The model under review builds one solid part; all positions refer to its coordinate system, in mm. A direction names the side the tool comes from. Coordinates: 2 decimals unless noted, no trailing zeros. Order: outer loops, then holes, each group sorted by start corner. A loop starts at its lowest first (then second) coordinate and runs counter-clockwise, first axis right, second up. Notation, with made-up numbers: M 79.25,70 L 97.25,70 A28 ccw 97.25,99 Z; hole C 26,16 d7. An arc over 180 degrees is marked long. Answer in a Markdown table with one row per item.
from build123d import *

# Parameters (mm, degrees)
F0_W     = 4.25
F0_H     = 4.25
F1_DEPTH = 5
F3_START = 2
F3_DEPTH = 4
F4_START = -2
F4_DEPTH = 4


# Not quite as in the source:
# - a feature names something its author has since deleted; it is built from what else it names


with BuildPart() as f1:
    # F0 (on Top) → F1 (new body, symmetric)
    with BuildSketch(Plane.XY):
        with BuildLine():
            Line((10.48, -5), (10.48, 5))
            Line((10.48, 5), (0.8137170322, 5))
            ThreePointArc((0.8137170322, 5), (1.6624848855, 2.5140482951), (1.95, -0.0970238614))
            ThreePointArc((1.95, -0.0970238614), (1.6852450978, -2.6038191253), (0.9026629175, -5))
            Line((0.9026629175, -5), (10.48, -5))
        make_face()
        with Locations((5.23, -0.25)):
            Rectangle(F0_W, F0_H, mode=Mode.SUBTRACT)
        with BuildLine():
            ThreePointArc((1.95, -0.0970238614), (1.6624848855, 2.5140482951), (0.8137170322, 5))
            Line((0.8137170322, 5), (0.48, 5))
            Line((0.48, 5), (0.48, -5))
            Line((0.48, -5), (0.9026629175, -5))
            ThreePointArc((0.9026629175, -5), (1.6852450978, -2.6038191253), (1.95, -0.0970238614))
        make_face()
        with BuildLine():
            Line((0.48, 5), (0.8137170322, 5))
            ThreePointArc((0.8137170322, 5), (-11.6370433083, 11.7975670747), (-21.8700390085, 1.9734055232))
            Line((-21.8700390085, 1.9734055232), (-20.3438487537, 1.9734055232))
            ThreePointArc((-20.3438487537, 1.9734055232), (-9.0096663788, 10.3513112192), (0.45, -0.0970238614))
            ThreePointArc((0.45, -0.0970238614), (-9.0810805838, -10.5522232935), (-20.3711800314, -2.0265944768))
            Line((-20.3711800314, -2.0265944768), (-21.89384892, -2.0265944768))
            ThreePointArc((-21.89384892, -2.0265944768), (-11.6020432417, -11.9962323131), (0.9026629175, -5))
            Line((0.9026629175, -5), (0.48, -5))
            Line((0.48, -5), (0.48, 5))
        make_face()
    extrude(amount=F1_DEPTH, both=True)

    # F2 (on Front) → F3 (join)
    with BuildSketch(Plane.XZ.offset(F3_START)):
        with BuildLine():
            Line((-28.1025181167, 1.8032137252), (-31.4321152449, 4.2247389093))
            Line((-31.4321152449, 4.2247389093), (-31.4321152449, -3.7752610907))
            Line((-31.4321152449, -3.7752610907), (-28.2350092218, -1.4500930739))
            ThreePointArc((-28.2350092218, -1.4500930739), (-28.8139991516, 0.2028375775), (-28.1025181167, 1.8032137252))
        make_face()
        with BuildLine():
            Line((-24.4076296068, 1.333455737), (-20.4321152449, 4.2247389093))
            Line((-20.4321152449, 4.2247389093), (-31.4321152449, 4.2247389093))
            Line((-31.4321152449, 4.2247389093), (-28.1025181167, 1.8032137252))
            ThreePointArc((-28.1025181167, 1.8032137252), (-26.1414263845, 2.4622306695), (-24.4076296068, 1.333455737))
        make_face()
        with BuildLine():
            Line((-20.4321152449, -3.7752610907), (-20.4321152449, 0.2247389093))
            Line((-20.4321152449, 0.2247389093), (-20.4321152449, 4.2247389093))
            Line((-20.4321152449, 4.2247389093), (-24.4076296068, 1.333455737))
            ThreePointArc((-24.4076296068, 1.333455737), (-24.1529758873, 0.7431613605), (-24.0659662098, 0.1061956755))
            ThreePointArc((-24.0659662098, 0.1061956755), (-24.128951902, -0.4371410894), (-24.3145681805, -0.9516589557))
            Line((-24.3145681805, -0.9516589557), (-20.4321152449, -3.7752610907))
        make_face()
        with BuildLine():
            Line((-31.4321152449, -3.7752610907), (-20.4321152449, -3.7752610907))
            Line((-20.4321152449, -3.7752610907), (-24.3145681805, -0.9516589557))
            ThreePointArc((-24.3145681805, -0.9516589557), (-26.1414263845, -2.2498393185), (-28.2350092218, -1.4500930739))
            Line((-28.2350092218, -1.4500930739), (-31.4321152449, -3.7752610907))
        make_face()
    extrude(amount=F3_DEPTH)

    # F2 (on Front) → F4 (join)
    with BuildSketch(Plane.XZ.offset(F4_START)):
        with BuildLine():
            Line((-28.1025181167, 1.8032137252), (-31.4321152449, 4.2247389093))
            Line((-31.4321152449, 4.2247389093), (-31.4321152449, -3.7752610907))
            Line((-31.4321152449, -3.7752610907), (-28.2350092218, -1.4500930739))
            ThreePointArc((-28.2350092218, -1.4500930739), (-28.8139991516, 0.2028375775), (-28.1025181167, 1.8032137252))
        make_face()
        with BuildLine():
            Line((-24.4076296068, 1.333455737), (-20.4321152449, 4.2247389093))
            Line((-20.4321152449, 4.2247389093), (-31.4321152449, 4.2247389093))
            Line((-31.4321152449, 4.2247389093), (-28.1025181167, 1.8032137252))
            ThreePointArc((-28.1025181167, 1.8032137252), (-26.1414263845, 2.4622306695), (-24.4076296068, 1.333455737))
        make_face()
        with BuildLine():
            Line((-20.4321152449, -3.7752610907), (-20.4321152449, 0.2247389093))
            Line((-20.4321152449, 0.2247389093), (-20.4321152449, 4.2247389093))
            Line((-20.4321152449, 4.2247389093), (-24.4076296068, 1.333455737))
            ThreePointArc((-24.4076296068, 1.333455737), (-24.1529758873, 0.7431613605), (-24.0659662098, 0.1061956755))
            ThreePointArc((-24.0659662098, 0.1061956755), (-24.128951902, -0.4371410894), (-24.3145681805, -0.9516589557))
            Line((-24.3145681805, -0.9516589557), (-20.4321152449, -3.7752610907))
        make_face()
        with BuildLine():
            Line((-31.4321152449, -3.7752610907), (-20.4321152449, -3.7752610907))
            Line((-20.4321152449, -3.7752610907), (-24.3145681805, -0.9516589557))
            ThreePointArc((-24.3145681805, -0.9516589557), (-26.1414263845, -2.2498393185), (-28.2350092218, -1.4500930739))
            Line((-28.2350092218, -1.4500930739), (-31.4321152449, -3.7752610907))
        make_face()
    extrude(amount=-F4_DEPTH)


solid = f1.part
(1) The part is to be moulded in two halves that separate along Y. For faces 1 (the flat face through (6, 5, 0)), 2 (the flat face through (1, 0, 5)), 3 (the flat face through (-29, 2, 0)), say which applies: +Y half, -Y half, draft (parallel to the pull), parting line (faces both ways), or undercut.
Report:
| item | result |
|---|---|
| face 1 | +Y half |
| face 2 | draft |
| face 3 | undercut |
(2) To check wall thickness, follow line 1 (Y direction, x = -10.05, z = -1.5); line 2 (Y direction, x = 6.5, z = -2) (3 decimals); line 3 (X direction, y = -0.5, z = -1.5) (3 decimals). State the ranges of each line that lie inside material, in increasing order. Write a range as [from, to].
Report:
| item | result |
|---|---|
| line 1 | [-12.1, -10.6], [10.4, 11.9] |
| line 2 | [-5, -2.375], [1.875, 5] |
| line 3 | [0.442, 3.105], [7.355, 10.48] |
(3) Insertion check: P1, Ø2.5, axis at x = -24.5, z = -1, coming from the +Y side; P2, Ø2, axis at x = 6, z = -1, coming from the +Y side; P3, Ø3, axis at x = -25.5, z = -1, coming from the -Y side. Each pin has a flat end and moves straight along its axis. Give the tip position at first contact, or say it passes through.
Report:
| item | result |
|---|---|
| P1 | y = 6 |
| P2 | y = 5 |
| P3 | y = -6 |
(4) Take a section at C-C (z = 3). Write out the cut boundary in (x, y) (3 decimals), then the cut area to 3 significant figures.
Report:
| item | result |
|---|---|
| outline | M -31.432,-6 L -20.498,-6 A12 ccw 0.903,-5 L 10.48,-5 L 10.48,5 L 0.814,5 A12 ccw -20.432,5.921 L -20.432,6 L -31.432,6 L -31.432,2 L -21.865,2 A12 ccw -21.87,1.973 L -20.344,1.973 A10.5 cw long -20.371,-2.027 L -20.432,-2.027 L -20.432,-2 L -31.432,-2 Z; hole M 3.105,-2.375 L 7.355,-2.375 L 7.355,1.875 L 3.105,1.875 Z |
| area | 252 mm^2 |
(5) Take a section at D-D (x = -27.5). Write out the cut boundary in (y, z), then the cut area to 3 significant figures.
Report:
| item | result |
|---|---|
| outline | M -6,-3.78 L -2,-3.78 L -2,-2.02 L -6,-2.02 Z; M -6,2.23 L -2,2.23 L -2,4.22 L -6,4.22 Z; M 2,-3.78 L 6,-3.78 L 6,-2.02 L 2,-2.02 Z; M 2,2.23 L 6,2.23 L 6,4.22 L 2,4.22 Z |
| area | 30.0 mm^2 |
(6) Machinability: for faces 4 (the flat face through (-24.8, -6, 2.1)), 5 (the flat face through (-24.8, -2, 2.1)), 6 (the flat face through (5, -2.375, 0)), which of the approach directions +Z, -Z, +X, -X, +Y, -Y give a long, thin tool a straight path to every point of the face, cutting with its end or side? Answer none if there is none.
Report:
| item | result |
|---|---|
| face 4 | +Z, -Z, -X, -Y |
| face 5 | +Z, -Z, -X |
| face 6 | +Z, -Z |
(7) Take a section at B-B (y = 8.75). Write out the cut boundary in (x, z), then the cut area to 3 significant figures.
Report:
| item | result |
|---|---|
| outline | M -18.16,-5 L -15.71,-5 L -15.71,5 L -18.16,5 Z; M -4.39,-5 L -1.94,-5 L -1.94,5 L -4.39,5 Z |
| area | 49.0 mm^2 |
(8) Take a section at A-A (x = -10.05). Write out the cut boundary in (y, z), then the cut area to 3 significant figures.
Report:
| item | result |
|---|---|
| outline | M -12.1,-5 L -10.6,-5 L -10.6,5 L -12.1,5 Z; M 10.4,-5 L 11.9,-5 L 11.9,5 L 10.4,5 Z |
| area | 30.0 mm^2 |
